Read the model definition and answer for the solid it produces. Units are mm, in the model's axes. Face numbers are marked on the shaded views. Round coordinates to 2 decimals unless told otherwise and drop trailing zeros. Loops run counter-clockwise (first coordinate to the right, second up) from the corner with the lowest first, then second, coordinate; pieces in that order, holes last. Notation, with made-up numbers: (16, 72.5) -> (30, 72.5) arc R27 cw to (30, 111.5) -> close; hole circle Ø11 at (-31.5, 75). An arc over 180 degrees is marked (long way). Put each result on its own line as item: value.
from build123d import *

# Parameters (mm, degrees)
SKETCH2_R               = 75.946
BOSS_EXTRUDE1_DEPTH     = 12.7
SKETCH3_R               = 5.55625
CUT_EXTRUDE1_DEPTH      = 1
CUT_EXTRUDE1_DEPTH_BACK = 13.7
CIRPATTERN2_COUNT       = 4
CIRPATTERN2_ANGLE       = 270
SKETCH11_R              = 69.596
CUT_EXTRUDE2_DEPTH      = 6.35


with BuildPart() as part:
    # Sketch2 → Boss-Extrude1 (new body)
    with BuildSketch(Plane(origin=(0, 0, 0), x_dir=(1, 0, 0), z_dir=(0, 1, 0))):
        Circle(SKETCH2_R)
    extrude(amount=BOSS_EXTRUDE1_DEPTH)

    # Sketch3 → Cut-Extrude1 (cut, two sides)
    with BuildSketch(Plane(origin=(0, 12.7, 0), x_dir=(1, 0, 0), z_dir=(0, 1, 0))) as cut_extrude1_sk:
        Circle(SKETCH3_R)
    extrude(amount=CUT_EXTRUDE1_DEPTH, mode=Mode.SUBTRACT)
    extrude(cut_extrude1_sk.sketch, amount=-CUT_EXTRUDE1_DEPTH_BACK, mode=Mode.SUBTRACT)

    # Sketch10 → 1_4-20 Tapped Hole1 (revolve, cut)
    with BuildSketch(Plane(origin=(-76.1746, 6.35, 0), x_dir=(0, 0, 1), z_dir=(0, 1, 0))):
        Polygon((0, 0), (0, 26.933816902), (2.5527, 25.4), (2.5527, 0), align=None)
    f_1_4_20_tapped_hole1 = revolve(axis=Axis((-82.5246, 6.35, 0), (1, 0, 0)), mode=Mode.SUBTRACT)

    # CirPattern2: 1_4-20 Tapped Hole1 ×4 about axis
    cirpattern2_axis = Axis((0, 12.7, 0), (0, -1, 0))
    for i in range(1, CIRPATTERN2_COUNT):
        add(f_1_4_20_tapped_hole1.rotate(cirpattern2_axis, i * CIRPATTERN2_ANGLE / (CIRPATTERN2_COUNT - 1)), mode=Mode.SUBTRACT)

    # Sketch11 → Cut-Extrude2 (cut)
    with BuildSketch(Plane.XZ):
        Circle(SKETCH11_R)
    extrude(amount=-CUT_EXTRUDE2_DEPTH, mode=Mode.SUBTRACT)


solid = part.part
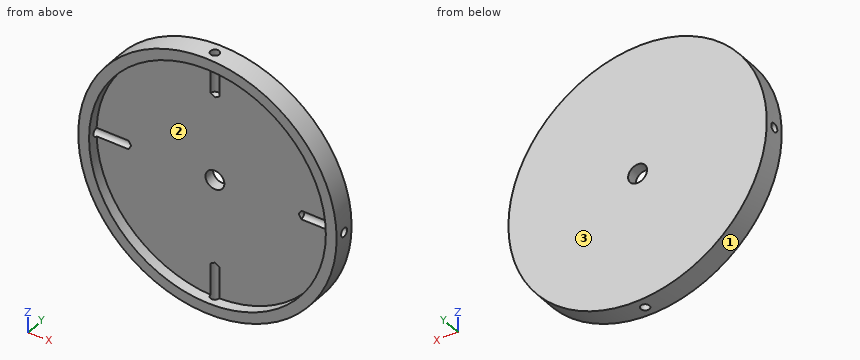
Item 1: Find the intervals of material crossed by line 1 along Y through (x, z) = (54.5, -6); line 2 along Y through (x, z) = (0, 59); line 3 along Z through (x, y) = (1, 2.5), in increasing order.
Derived:
line 1: y = 6.35 to 12.7
line 2: y = 8.9 to 12.7
line 3: z = -75.94 to -69.59, 69.59 to 75.94
Item 2: Flat-ended cylindrical pins translate along their axes: pin 1 Ø6.5 at (x, y) = (0, 6.35) entering from -Z; pin 2 Ø1.5 at (x, z) = (17, 35) entering from -Y; pin 3 Ø2 at (y, z) = (7, -2.5) entering from +X; pin 4 Ø4 at (y, z) = (6.35, 0) entering from +X. Find the tip coordinate at first contact, or state that the pin passes through.
Derived:
pin 1: stops at z = -75.95
pin 2: stops at y = 6.35
pin 3: stops at x = 75.92
pin 4: stops at x = 50.44
Item 3: The part is cut by section A-A (x = 0). Determine the outline of the cut face in (y, z), then the cut area to 3 significant figures.
Derived:
outline: (0, -75.95) -> (3.8, -75.95) -> (3.8, -69.6) -> (0, -69.6) -> close; (0, 69.6) -> (3.8, 69.6) -> (3.8, 75.95) -> (0, 75.95) -> close; (6.35, -49.24) -> (8.9, -50.77) -> (8.9, -75.95) -> (12.7, -75.95) -> (12.7, -5.56) -> (6.35, -5.56) -> close; (6.35, 5.56) -> (12.7, 5.56) -> (12.7, 75.95) -> (8.9, 75.95) -> (8.9, 50.77) -> (6.35, 49.24) -> close
area: 810 mm^2
Item 4: The part is cut by section C-C (z = 17). Determine the outline of the cut face in (x, y), then the cut area to 3 significant figures.
Derived:
outline: (-74.02, 0) -> (-67.49, 0) -> (-67.49, 6.35) -> (67.49, 6.35) -> (67.49, 0) -> (74.02, 0) -> (74.02, 12.7) -> (-74.02, 12.7) -> close
area: 1,020 mm^2
Item 5: The part is cut by section D-D (x = 66). Determine the outline of the cut face in (y, z).
Derived:
outline: (0, -37.57) -> (12.7, -37.57) -> (12.7, 37.57) -> (0, 37.57) -> (0, 22.08) -> (6.35, 22.08) -> (6.35, 2.55) arc R2.55 cw to (6.35, -2.55) -> (6.35, -22.08) -> (0, -22.08) -> close
Item 6: For a pull along X with two mould halves and no side action, classify the marked faces 1, 2 and 3 as pulls with the +X half, pulls with the -X half, needs draft (parallel to the pull), parting line crosses it, or undercut.
Derived:
face 1: parting line crosses it
face 2: undercut
face 3: needs draft
Item 7: The part is cut by section B-B (z = 0). Determine the outline of the cut face in (x, y).
Derived:
outline: (-75.95, 0) -> (-69.6, 0) -> (-69.6, 3.8) -> (-75.95, 3.8) -> close; (-75.95, 8.9) -> (-50.77, 8.9) -> (-49.24, 6.35) -> (-5.56, 6.35) -> (-5.56, 12.7) -> (-75.95, 12.7) -> close; (5.56, 6.35) -> (49.24, 6.35) -> (50.77, 8.9) -> (75.95, 8.9) -> (75.95, 12.7) -> (5.56, 12.7) -> close; (69.6, 0) -> (75.95, 0) -> (75.95, 3.8) -> (69.6, 3.8) -> close
